Input: part model. Units: mm. Frame: model coordinates. Face numbers are marked on the shaded views. A direction names the side the tool comes from. Give positions to 0.01 mm unless a question says otherwise; leave off trailing zeros. Order: outer loops, then holes, each group sorted by start corner. A loop starts at its lowest first (then second) coordinate and runs counter-clockwise, first axis right, second up. Notation, with made-up numbers: (38.25, 39) -> (65.25, 39) arc R22 ccw to (65.25, 67) -> close; hole circle Ø10 at (6.25, 68.25). An arc over 180 degrees is marked (long way). Use a Markdown table: item, result. Add a question column.
Autodesk Inventor part; units mm, degrees
ref_plane "YZ Plane" through (0, 0, 0) normal (1, 0, 0) x (0, 1, 0)
ref_plane "XZ Plane" through (0, 0, 0) normal (0, 1, 0) x (-1, 0, 0)
ref_plane "XY Plane" through (0, 0, 0) normal (0, 0, 1) x (1, 0, 0)
sketch "Sketch1" plane through (0, 0, 0) normal (0, 1, 0) x (-1, 0, 0)
  line L0 (34, 0) -> (64.4, 0) construction
  line L1 (34, 32) -> (36, 32) construction
  line L2 (34, 91) -> (34, 97)
  line L3 (34, 97) -> (34, 91)
  line L4 (34, 91) -> (35.4142, 89.5858)
  line L5 (35.4142, 89.5858) -> (35.4142, 89.5858)
  line L6 (35.4142, 89.5858) -> (35.4142, 33.4142)
  line L7 (34, 97) -> (39, 97)
  line L8 (34, 97) -> (39, 97) construction
  line L9 (39, 97) -> (39, 129)
  line L10 (39, 129) -> (36, 129)
  line L11 (36, 129) -> (36, 144)
  line L12 (33.9171, 144) -> (36, 144)
  line L13 (31.9171, 142) -> (31.9171, 125.958)
  line L14 (31.9171, 144) -> (47.9592, 144) construction
  line L15 (31.9171, 125.958) -> (34.7455, 123.1296)
  line L16 (31.9171, 125.958) -> (35.9171, 125.958) construction
  line L17 (34.7455, 123.1296) -> (34.7455, 118.1296)
  line L18 (34.7455, 118.1296) -> (26.9171, 118.1296)
  line L19 (26.9171, 118.1296) -> (25.1856, 115.1305)
  line L20 (26.9171, 118.1296) -> (30.3802, 118.1296) construction
  line L21 (25.1856, 42.2286) -> (28.1856, 37.0325)
  line L22 (25.1856, 42.2286) -> (31.1856, 42.2286) construction
  line L23 (28.1856, 37.0325) -> (28.1856, 1.6)
  line L24 (32.4, 0) -> (29.7856, 0)
  line L25 (28.1856, 1.6) -> (29.7856, 0)
  line L26 (34, 1.6) -> (32.4, 0)
  line L27 (33.9171, 144) -> (31.9171, 142)
  line L28 (33.9, 14.92) -> (32.5, 14.92)
  line L29 (32.4, 14.82) -> (32.4, 10.32)
  line L30 (32.5, 10.22) -> (33.9, 10.22)
  line L31 (34, 1.6) -> (34, 10.12)
  arc A0 (32.5, 14.92) -> (32.4, 14.82) centre (32.5, 14.82) ccw
  arc A1 (32.4, 10.32) -> (32.5, 10.22) centre (32.5, 10.32) ccw
  arc A2 (33.9, 14.92) -> (34, 15.02) centre (33.9, 15.02) ccw
  arc A3 (34, 10.12) -> (33.9, 10.22) centre (33.9, 10.12) ccw
  line L32 (34, 15.02) -> (34, 32)
  line L33 (34, 32) -> (35.4142, 33.4142)
  line L34 (25.1856, 115.1305) -> (25.1856, 42.2286)
  line L35 (0, -28.8) -> (0, 172.8001)
  point P0 (0, 0)
  point P1 (28.1856, 0)
  point P2 (32.4, 14.92)
  point P3 (32.4, 10.22)
  dimension "d2" = 32
  dimension "d4" = 2
  dimension "d8" = 65
  dimension "d12" = 5
  dimension "d14" = 32
  dimension "d16" = 90
  dimension "d18" = 90
  dimension "d22" = 90
  dimension "d23" = 4
  dimension "d24" = 45
  dimension "d25" = 5
  dimension "d26" = 135
  dimension "d28" = 120
  dimension "d30" = 6
  dimension "d31" = 60
  dimension "d32" = 150
  dimension "d33" = 1.6
  dimension "d34" = 1.6
  dimension "d35" = 1.6
  dimension "d36" = 1.6
  dimension "d37" = 2
  dimension "d38" = 2
  dimension "d39" = 4.7
  dimension "d41" = 90
  dimension "d42" = 0.1
revolve "Revolution1" add sketch "Sketch1" angle 360 about axis through (0, 0, -10) along (0, 0, 1)
thread "Thread1"
thread "Thread2"
sketch "Sketch2" plane through (0, 0, 144) normal (0, 0, 1) x (1, 0, 0)
  line L0 (29.1771, -25.8785) -> (7.8229, -38.2074)
  line L1 (-7.8229, -38.2074) -> (-29.1771, -25.8785)
  line L2 (-37, -12.3288) -> (-37, 12.3288)
  line L3 (-29.1771, 25.8785) -> (-7.8229, 38.2074)
  line L4 (7.8229, 38.2074) -> (29.1771, 25.8785)
  line L5 (37, 12.3288) -> (37, -12.3288)
  arc A0 (29.1771, -25.8785) -> (37, -12.3288) centre (0, 0) ccw
  arc A1 (37, 12.3288) -> (29.1771, 25.8785) centre (0, 0) ccw
  arc A2 (7.8229, 38.2074) -> (-7.8229, 38.2074) centre (0, 0) ccw
  arc A3 (-29.1771, 25.8785) -> (-37, 12.3288) centre (0, 0) ccw
  arc A4 (-37, -12.3288) -> (-29.1771, -25.8785) centre (0, 0) ccw
  arc A5 (-7.8229, -38.2074) -> (7.8229, -38.2074) centre (0, 0) ccw
  circle A6 centre (0, 0) radius 36
  dimension "d48" = 74
extrude "Extrusion1" add sketch "Sketch2" against normal blind 47
equation "\"d35\" = d33"
equation "\"d36\" = d35"
equation "\"d38\" = d37"
properties part number "Переводник"
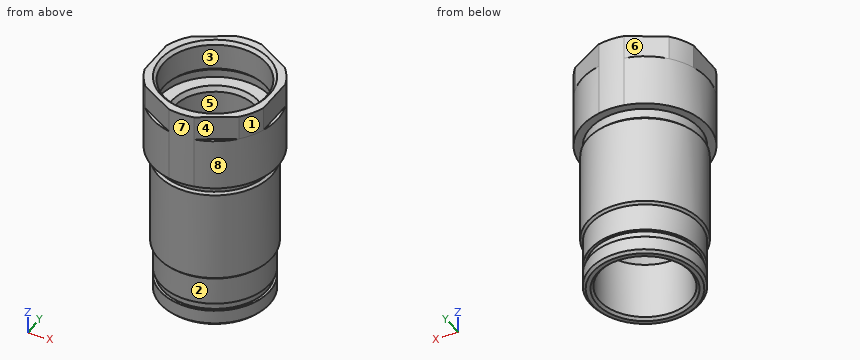
Q1. Draft query along X for the marked faces 5, 6, 7 and 8. Return one class per face: +X half, -X half, draft (parallel to the pull), parting line (faces both ways), or undercut.
Q2. Ray query, line 1 (X direction, y = 0, z = 21); line 2 (X direction, y = 0, z = 69); line 3 (Z direction, x = -22, y = 24.5). Return the intervals inside material, ascending.
Q3. Section query B-B (z = 62). Return loops of the section in (x, y).
Q4. Access query for the marked faces 1, 2, 3 and 4. Directions: +Z, -Z, +X, -X, +Y, -Y. A direction counts if a zero-diameter tool reaches every point of the face in a straight line with its end or side. Return the directions, or none.
Q5. First-contact query: pin 1 (4.5 mm diameter, centred on y = 0, z = 137, fed in from +X); pin 2 (8 mm diameter, centred on x = 8.5, z = 19, fed in from +Y); pin 3 (10 mm diameter, centred on x = 19, y = 33, fed in from +Z); pin 4 (6 mm diameter, centred on y = 29, z = 128.5, fed in from -X). Flat tips, straight axial feed; report the tip coordinate or a pass-through.
Solution:
| question | item | result |
|---|---|---|
| 1 | face 5 | undercut |
| 1 | face 6 | -X half |
| 1 | face 7 | parting line |
| 1 | face 8 | +X half |
| 2 | line 1 | x = -34 to -28.19, 28.19 to 34 |
| 2 | line 2 | x = -35.41 to -25.19, 25.19 to 35.41 |
| 2 | line 3 | z = 0.53 to 10.22, 14.92 to 118.13, 124.95 to 143.01 |
| 3 | outline | circle Ø70.83 at (0, 0); hole circle Ø50.37 at (0, 0) |
| 4 | face 1 | +Z, -Z, +X, -Y |
| 4 | face 2 | -Z |
| 4 | face 3 | +Z |
| 4 | face 4 | +Z, +X, -Y |
| 5 | pin 1 | stops at x = 37 |
| 5 | pin 2 | stops at y = 33.7 |
| 5 | pin 3 | stops at z = 144 |
| 5 | pin 4 | stops at x = -29.07 |
